Answer from the drawing. Dimensions are ordinates in mm from the lowest x, y and z of the part. A direction names the side the tool comes from. Coordinates: 2 decimals unless noted, no trailing zeros. Order: outer loops, then holes, each group sorted by start corner. A loop starts at its lowest first (then second) coordinate and runs counter-clockwise, first axis right, second up. Notation, with made-up numbers: M 78.5,-11.5 L 83.5,-11.5 A26 cw 83.5,14.5 Z; hole C -4,19.25 d8. An arc over 180 degrees is marked long. Use a Markdown table: item, result.
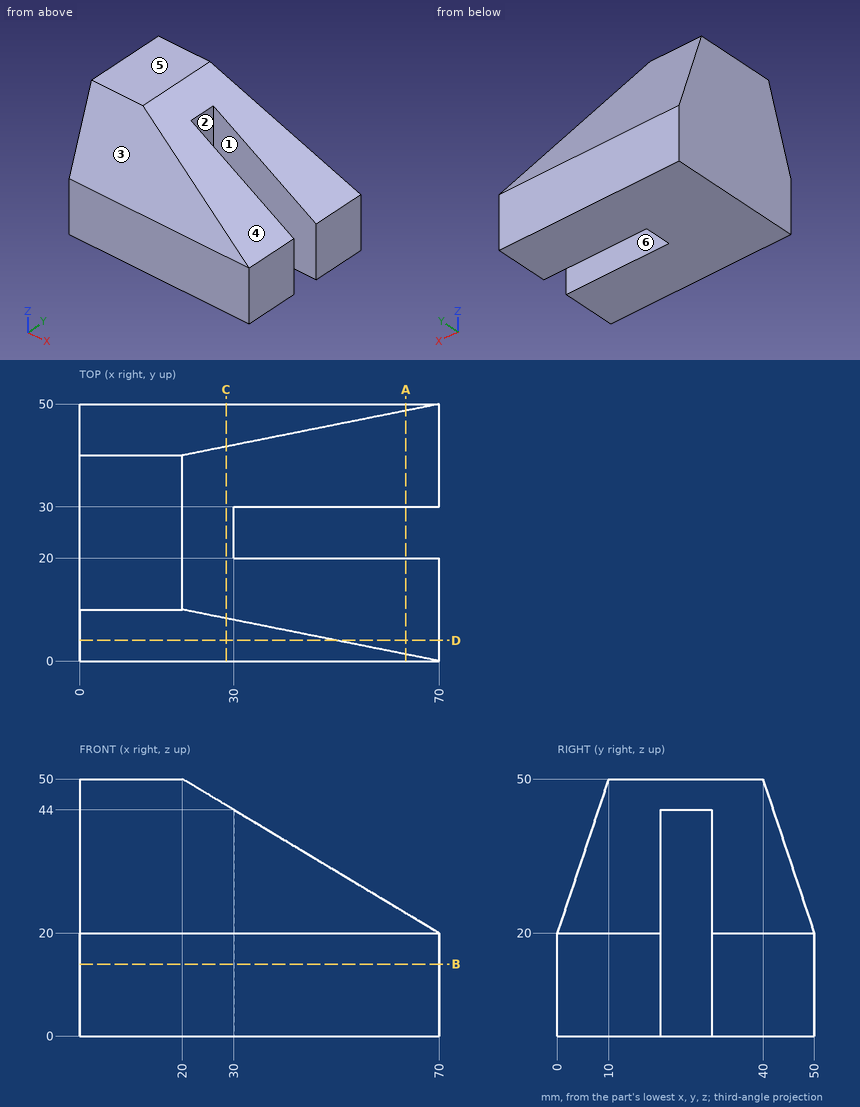
(1) A cutting plane is placed at C-C (x = 28.5). Determine the outline of the cut face in (y, z).
Conclusion:
| item | result |
|---|---|
| outline | M 0,0 L 50,0 L 50,20 L 41.7,44.9 L 8.3,44.9 L 0,20 Z |
(2) Given P1, Ø10, axis at x = 29.5, z = 26, coming from the -Y side; P2, Ø3, axis at y = 8.5, z = 23, coming from the +X side; P3, Ø8, axis at y = 25, z = 31.5, coming from the +X side; P4, Ø8, axis at x = 56, z = 35.5, coming from the +Y side, each flat-ended and moving along its own axis, determine where each tip first touches the part or whether it passes through.
Conclusion:
| item | result |
|---|---|
| P1 | y = 0.33 |
| P2 | x = 67.5 |
| P3 | x = 30 |
| P4 | through |
(3) Which of the six approach directions +Z, -Z, +X, -X, +Y, -Y give full straight-line access (tool end or side, diameter ignored) to the marked faces 5 and 6?
Conclusion:
| item | result |
|---|---|
| face 5 | +Z, +X, -X, +Y, -Y |
| face 6 | +Z, -Z, +X |
(4) A cutting plane is placed at B-B (z = 14). Determine the outline of the cut face in (x, y).
Conclusion:
| item | result |
|---|---|
| outline | M 0,0 L 70,0 L 70,20 L 30,20 L 30,30 L 70,30 L 70,50 L 0,50 Z |
(5) A cutting plane is placed at A-A (x = 63.5). Determine the outline of the cut face in (y, z), then the cut area to 3 significant figures.
Conclusion:
| item | result |
|---|---|
| outline | M 0,0 L 20,0 L 20,23.9 L 1.3,23.9 L 0,20 Z; M 30,0 L 50,0 L 50,20 L 48.7,23.9 L 30,23.9 Z |
| area | 951 mm2 |
(6) Determine the mould class of the marked faces 1, 2, 3 and 4 for opening direction Y: pulls with the +Y half, pulls with the -Y half, needs draft (parallel to the pull), parting line crosses it, or undercut.
Conclusion:
| item | result |
|---|---|
| face 1 | undercut |
| face 2 | undercut |
| face 3 | pulls with the -Y half |
| face 4 | needs draft |
(7) A cutting plane is placed at D-D (y = 4). Determine the outline of the cut face in (x, z).
Conclusion:
| item | result |
|---|---|
| outline | M 0,0 L 70,0 L 70,20 L 50,32 L 0,32 Z |
(8) Straight lines are drawn through the part: L1, parallel to Y at x = 44.5, z = 19; L2, parallel to X at y = 25, z = 32.5; L3, parallel to Z at x = 25, y = 17. For each, find the intervals that lie inside material, in ascending order.
Conclusion:
| item | result |
|---|---|
| L1 | 0 to 20, 30 to 50 |
| L2 | 0 to 30 |
| L3 | 0 to 47 |
